```python
from build123d import *

# Parameters (mm, degrees)
SKETCH1_W           = 79
SKETCH1_H           = 64
BOSS_EXTRUDE1_DEPTH = 4
BOSS_EXTRUDE2_DEPTH = 15
SKETCH3_W           = 7
SKETCH3_H           = 6
BOSS_EXTRUDE3_DEPTH = 3
CUT_EXTRUDE1_DEPTH  = 4
BOSS_EXTRUDE4_DEPTH = 4
FILLET1_R           = 2
FILLET2_R           = 5
FILLET3_R           = 4


with BuildPart() as part:
    # Sketch1 → Boss-Extrude1 (new body)
    with BuildSketch(Plane.XY):
        with Locations((36.5, 29)):
            Rectangle(SKETCH1_W, SKETCH1_H)
    extrude(amount=BOSS_EXTRUDE1_DEPTH)

    # Sketch2 → Boss-Extrude2 (add)
    with BuildSketch(Plane.XY.offset(4)):
        Polygon((76, -3), (76, 3), (73, 3), (73, 0), (69, 0), (69, -3), align=None)
        Polygon((0, 3), (-3, 3), (-3, -3), (4, -3), (4, 0), (0, 0), align=None)
        Polygon((0, 58), (4, 58), (4, 61), (-3, 61), (-3, 55), (0, 55), align=None)
        Polygon((76, 61), (69, 61), (69, 58), (73, 58), (73, 55), (76, 55), align=None)
    extrude(amount=BOSS_EXTRUDE2_DEPTH)

    # Sketch3 → Boss-Extrude3 (add)
    with BuildSketch(Plane.XY.offset(19)):
        with Locations((0.5, 58)):
            Rectangle(SKETCH3_W, SKETCH3_H)
        with Locations((0.5, 0)):
            Rectangle(SKETCH3_W, SKETCH3_H)
        with Locations((72.5, 0)):
            Rectangle(SKETCH3_W, SKETCH3_H)
        with Locations((72.5, 58)):
            Rectangle(SKETCH3_W, SKETCH3_H)
    extrude(amount=BOSS_EXTRUDE3_DEPTH)

    # Sketch4 → Cut-Extrude1 (cut)
    with BuildSketch(Plane(origin=(0, 0, 0), x_dir=(-1, 0, 0), z_dir=(0, 0, -1))):
        Polygon((3, 27.803812192), (-8.289774189, 13.867997178), (0.187909827, 7), (3, 7), align=None)
        Polygon((-73.187909827, 7), (-64.710225811, 13.867997178), (-76, 27.803812192), (-76, 7), align=None)
        Polygon((-7, 51), (-66, 51), (-66, 28.65625), (-58.25574912, 19.09694032), (-36.5, 29), (-14.74425088, 19.09694032), (-7, 28.65625), align=None)
        with BuildLine():
            Line((-66, -2.620585177), (-66, -3))
            Line((-66, -3), (-7, -3))
            Line((-7, -3), (-7, -2.620585177))
            Line((-7, -2.620585177), (-29.594686034, 15.683970598))
            ThreePointArc((-29.594686034, 15.683970598), (-36.5, 14), (-43.405313966, 15.683970598))
            Line((-43.405313966, 15.683970598), (-66, -2.620585177))
        make_face()
    extrude(amount=-CUT_EXTRUDE1_DEPTH, mode=Mode.SUBTRACT)

    # Sketch5 → Boss-Extrude4 (add)
    with BuildSketch(Plane(origin=(0, 0, 0), x_dir=(-1, 0, 0), z_dir=(0, 0, -1))):
        Polygon((-24.697125845, 61), (-32.5, 73), (-40.5, 73), (-48.302874155, 61), align=None)
        with BuildLine():
            Line((-38.826625292, 69.61473034), (-36.5, 71.5))
            Line((-36.5, 71.5), (-34.173374708, 69.61473034))
            ThreePointArc((-34.173374708, 69.61473034), (-36.5, 63.5), (-38.826625292, 69.61473034))
        make_face(mode=Mode.SUBTRACT)
    extrude(amount=-BOSS_EXTRUDE4_DEPTH)

    # Fillet1
    fillet1_edges = [part.edges().sort_by_distance(p)[0] for p in [
        (4, 1.5, 19),
        (69, 3, 20.5),
        (69, 55, 20.5),
        (32.5, 73, 2),
        (24.697125845, 61, 2),
        (48.302874155, 61, 2),
        (40.5, 73, 2),
        (76, 61, 11),
        (76, -3, 11),
        (-3, -3, 11),
        (-3, 61, 11),
        (4, 55, 20.5),
    ]]
    fillet(fillet1_edges, radius=FILLET1_R)

    # Fillet2
    fillet2_edges = [part.edges().sort_by_distance(p)[0] for p in [
        (76, 27.803812192, 2),
        (64.710225811, 13.867997178, 2),
        (-3, 27.803812192, 2),
        (8.289774189, 13.867997178, 2),
        (7, 28.65625, 2),
        (14.74425088, 19.09694032, 2),
        (36.5, 29, 2),
        (58.25574912, 19.09694032, 2),
        (66, 28.65625, 2),
        (43.405313966, 15.683970598, 2),
        (29.594686034, 15.683970598, 2),
    ]]
    fillet(fillet2_edges, radius=FILLET2_R)

    # Fillet3
    # the kernel refuses this fillet: 4 mm, written as the material it takes off along each edge
    with BuildSketch(Plane(origin=(76, 7, -9.548844905), x_dir=(-1, 0, 0), z_dir=(0, 0, 1))) as fillet3_piece_1:
        with BuildLine():
            CenterArc((4, 3.819537962), FILLET3_R, 180, 72.723847708)
            Line((0, 3.819537962), (-0.08, 3.819537962))
            Line((-0.08, 3.819537962), (-0.08, 0))
            Line((-0.08, 0), (0, -0.08))
            ThreePointArc((0, -0.08), (1.406045086, -0.08), (2.788331976, -0.076390759))
            Line((2.788331976, -0.076390759), (2.812090173, 0))
        make_face()
    extrude(amount=23.097689809, mode=Mode.SUBTRACT)
    with BuildSketch(Plane(origin=(-3, 7, -9.548844905), x_dir=(1, 0, 0), z_dir=(0, 0, 1))) as fillet3_piece_2:
        with BuildLine():
            CenterArc((4, -3.819537962), FILLET3_R, 107.276152292, 72.723847708)
            Line((0, -3.819537962), (-0.08, -3.819537962))
            Line((-0.08, -3.819537962), (-0.08, 0))
            Line((-0.08, 0), (0, 0.08))
            ThreePointArc((0, 0.08), (1.406045086, 0.08), (2.788331976, 0.076390759))
            Line((2.788331976, 0.076390759), (2.812090173, 0))
        make_face()
    extrude(amount=23.097689809, mode=Mode.SUBTRACT)
    with BuildSketch(Plane(origin=(7, -3, -4.251002073), x_dir=(0, 1, 0), z_dir=(0, 0, 1))) as fillet3_piece_3:
        with BuildLine():
            CenterArc((4, 1.700400829), FILLET3_R, 180, 25.15700637)
            Line((0, 1.700400829), (-0.08, 1.700400829))
            Line((-0.08, 1.700400829), (-0.08, 0))
            Line((-0.08, 0), (0, -0.08))
            ThreePointArc((0, -0.08), (0.189707412, -0.08), (0.30700312, -0.034008017))
            Line((0.30700312, -0.034008017), (0.379414823, 0))
        make_face()
    extrude(amount=12.502004146, mode=Mode.SUBTRACT)
    with BuildSketch(Plane(origin=(66, -3, -4.251002073), x_dir=(1, 0, 0), z_dir=(0, 0, 1))) as fillet3_piece_4:
        with BuildLine():
            CenterArc((1.700400829, 4), FILLET3_R, 244.84299363, 25.15700637)
            Line((0, 0.379414823), (-0.034008017, 0.30700312))
            ThreePointArc((-0.034008017, 0.30700312), (-0.08, 0.189707412), (-0.08, 0))
            Line((-0.08, 0), (0, -0.08))
            Line((0, -0.08), (1.700400829, -0.08))
            Line((1.700400829, -0.08), (1.700400829, 0))
        make_face()
    extrude(amount=12.502004146, mode=Mode.SUBTRACT)


solid = part.part
```
Design review of the part built by this model. Coordinates are the model's own, in mm. A direction names the side the tool comes from. Give positions to 0.01 mm unless a question says otherwise; leave off trailing zeros. Loops run counter-clockwise (first coordinate to the right, second up) from the corner with the lowest first, then second, coordinate; pieces in that order, holes last. Notation, with made-up numbers: M 28.5,11.5 L 41.5,11.5 A32 ccw 41.5,37.5 Z; hole C 10.5,81.25 d8. An arc over 180 degrees is marked long. Return JSON: item names as keys, results as strings. Group by question number.
Item 1: Insertion check: pin 1 Ø10 at (x, z) = (60.5, 10.5) entering from +Y; pin 2 Ø10 at (x, z) = (5.5, 3) entering from +Y; pin 3 Ø1.2 at (y, z) = (60, 14.5) entering from -X; pin 4 Ø5 at (x, y) = (45.5, 25) entering from +Z. Each pin has a flat end and moves straight along its axis. Give the tip position at first contact, or say it passes through.
Item 2: For probe 1 along Y at (x, z) = (36.5, 1.4); probe 2 along X at (y, z) = (38, 1); probe 3 along Y at (x, z) = (38, 1.25), list the stretches that pass through material, from the lowest coordinate up.
Item 3: Mouldability with a two-part tool opening along Z and no side actions: class faces 5 (the flat face through (1, 2, 19)), 6 (the flat face through (75, 3, 13)) as released by +Z, released by -Z, zero draft, split by the parting line, or undercut.
Item 4: We need section B-B (z = 12). Give the boundary of the cut face in (x, y), and give its area (3 significant figures).
Item 5: We need section C-C (x = 43.5). Give the boundary of the cut face in (y, z).
Item 6: Tool access review of faces 1 (the flat face through (37.68, 70.544, 1.972)), 2 (the cylindrical face through (69.57, 55.6, 20.52)), 3 (the cylindrical face through (75.242, 5.523, 1.972)), 4 (the flat face through (-2, 55, 13)): name each direction out of +Z, -Z, +X, -X, +Y, -Y from which nothing blocks a thin tool from reaching the whole face with its end or side.
Item 7: We need section A-A (y = 35.5). Give the boundary of the cut face in (x, z).
Output:
{
 "1": {"pin 1": "passes through", "pin 2": "stops at y = 61", "pin 3": "stops at x = -2.96", "pin 4": "stops at z = 4"},
 "2": {"probe 1": "y = 14 to 28.51, 51 to 63.5, 71.5 to 73", "probe 2": "x = -3 to 7, 66 to 76", "probe 3": "y = 14.08 to 28.28, 51 to 63.84, 70.28 to 73"},
 "3": {"face 5": "undercut", "face 6": "zero draft"},
 "4": {"outline": "M -3,-1 A2 ccw -1,-3 L 4,-3 L 4,0 L 0,0 L 0,3 L -3,3 Z; M -3,55 L 0,55 L 0,58 L 4,58 L 4,61 L -1,61 A2 ccw -3,59 Z; M 69,-3 L 74,-3 A2 ccw 76,-1 L 76,3 L 73,3 L 73,0 L 69,0 Z; M 69,58 L 73,58 L 73,55 L 76,55 L 76,59 A2 ccw 74,61 L 69,61 Z", "area": "117 mm^2"},
 "5": {"outline": "M 14.85,0 L 25.81,0 L 25.81,4 L 14.85,4 Z; M 51,0 L 68.39,0 L 68.39,4 L 51,4 Z"},
 "6": {"face 1": "+Z, -Z", "face 2": "+Z", "face 3": "+Z, -Z, +X", "face 4": "+Z, +X, -X"},
 "7": {"outline": "M -3,0 L 7,0 L 7,4 L -3,4 Z; M 66,0 L 76,0 L 76,4 L 66,4 Z"}
}
